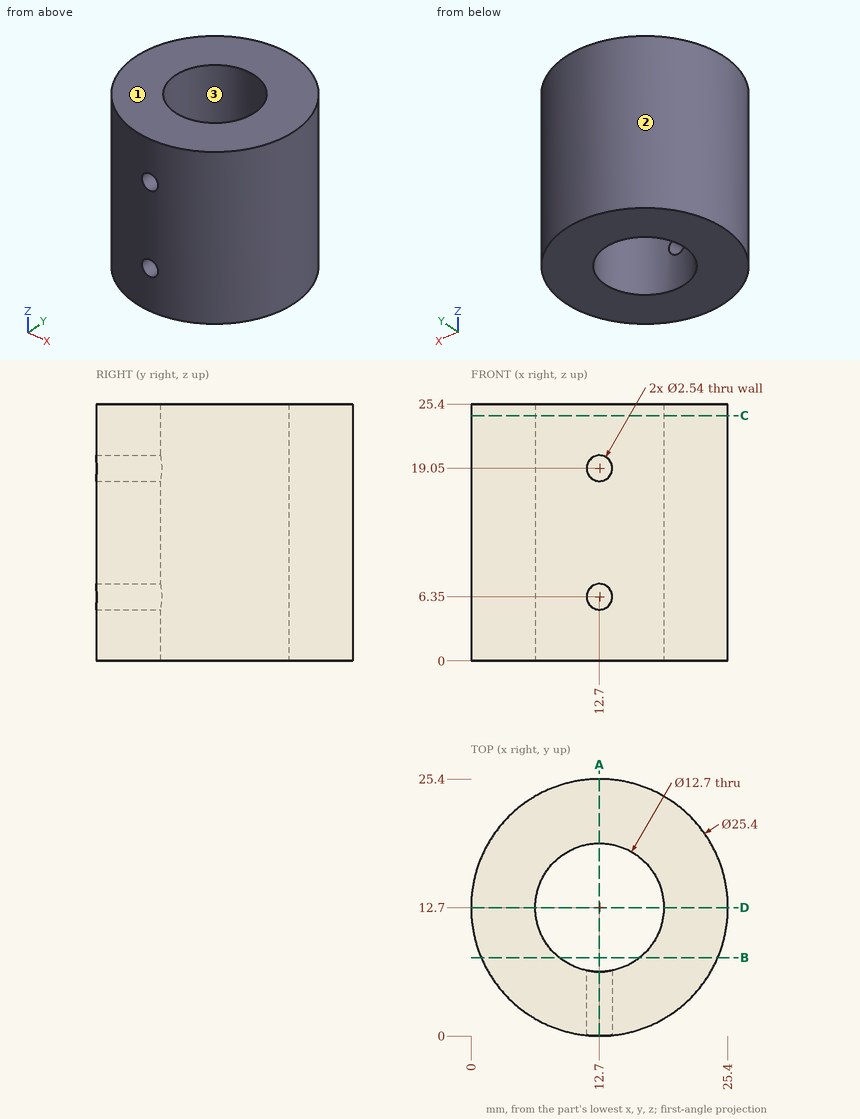
Here's the drawing with two shaded views (mm, measured from the low corner). I have some questions. Give positions to 0.01 mm unless a question says otherwise; leave off trailing zeros. Order: outer loops, then holes, each group sorted by start corner. A loop starts at its lowest first (then second) coordinate and runs counter-clockwise, first axis right, second up. Notation, with made-up numbers: M 38.5,-38 L 61.5,-38 A17 cw 61.5,-22 Z; hole C 73,-4.5 d9. An arc over 180 degrees is marked long. One line per question, with ' | ' between items.
Item 1: Suppose I cut it at D-D, the plane y = 12.7. Write out the boundary of the cut face in (x, z).
Answer block:
outline: M 0,0 L 6.35,0 L 6.35,25.4 L 0,25.4 Z; M 19.05,0 L 25.4,0 L 25.4,25.4 L 19.05,25.4 Z
Item 2: Suppose I cut it at C-C, the plane z = 24.25. Write out the boundary of the cut face in (x, y), then the cut area to 3 significant figures.
Answer block:
outline: C 12.7,12.7 d25.4; hole C 12.7,12.7 d12.7 | area: 380 mm2
Item 3: We'd pull the mould along X, two halves only. Please class the marked faces 1, 2 and 3: released by +X, released by -X, zero draft, split by the parting line, or undercut.
Answer block:
face 1: zero draft | face 2: split by the parting line | face 3: undercut
Item 4: I'm going to push flat-ended pins straight in: pin 1 Ø2 at (y, z) = (11, 21.5) entering from -X; pin 2 Ø2 at (y, z) = (18, 3.5) entering from -X; pin 3 Ø5 at (y, z) = (21, 14) entering from +X; pin 4 Ø11.5 at (x, y) = (12.7, 12.7) entering from +Z. Where does each tip first touch, or does it pass through?
Answer block:
pin 1: stops at x = 0.02 | pin 2: stops at x = 0.75 | pin 3: stops at x = 24 | pin 4: passes through
Item 5: Suppose I cut it at B-B, the plane y = 7.75. Write out the boundary of the cut face in (x, z).
Answer block:
outline: M 1,0 L 8.72,0 L 8.72,25.4 L 1,25.4 Z; M 16.68,0 L 24.4,0 L 24.4,25.4 L 16.68,25.4 Z
Item 6: Suppose I cut it at A-A, the plane x = 12.7. Write out the boundary of the cut face in (y, z).
Answer block:
outline: M 0,0 L 6.35,0 L 6.35,5.08 L 0,5.08 Z; M 0,7.62 L 6.35,7.62 L 6.35,17.78 L 0,17.78 Z; M 0,20.32 L 6.35,20.32 L 6.35,25.4 L 0,25.4 Z; M 19.05,0 L 25.4,0 L 25.4,25.4 L 19.05,25.4 Z
Item 7: Please list where these lines run through material, in increasing order: L1, parallel to Z at x = 12.7, y = 4.5; L2, parallel to Y at x = 12.7, z = 12; L3, parallel to Y at x = 14.75, z = 12.75.
Answer block:
L1: z = 0 to 5.08, 7.62 to 17.78, 20.32 to 25.4 | L2: y = 0 to 6.35, 19.05 to 25.4 | L3: y = 0.17 to 6.69, 18.71 to 25.23
